from build123d import *

# Parameters (mm, degrees)
F0_R     = 6.5
F0_R_2   = 2.15
F1_DEPTH = 1
F2_R     = 0.49999


# Not quite as in the source:
# - a fillet or chamfer is up to 0.001 mm smaller than in the source, because OpenCascade refuses the exact size


with BuildPart() as f1:
    # F0 (on Top) → F1 (new body)
    with BuildSketch(Plane.XY):
        Circle(F0_R)
        Circle(F0_R_2, mode=Mode.SUBTRACT)
    extrude(amount=F1_DEPTH)

    # F2 (radius 0.5 in the source; OpenCascade refuses exactly that, so slightly less here)
    f2_edges = [f1.edges().sort_by_distance(p)[0] for p in [
        (-6.5, 0, 1),
        (-2.15, 0, 1),
        (6.5, 0, 0.5),
        (-6.5, 0, 0),
        (-2.15, 0, 0),
        (2.15, 0, 0.5),
    ]]
    fillet(f2_edges, radius=F2_R)


solid = f1.part
Can you work these out from the model? Positions are in its coordinate system, mm. Round coordinates to 2 decimals unless told otherwise and drop trailing zeros. Loops run counter-clockwise (first coordinate to the right, second up) from the corner with the lowest first, then second, coordinate; pieces in that order, holes last. Notation, with made-up numbers: (-20, 37) - (-8, 37) arc R21 cw to (-8, 61) - close; hole circle Ø10 at (-28, 54.5). An arc over 180 degrees is marked (long way). Use CSV: the item, a comma, the result in double quotes. Start each with the question number.
1) If we section it at C-C on z = 0.65: Write out the boundary of the cut face in (x, y).
2) Please list where these lines run through material, in increasing order: probe 1 along Y at (x, z) = (0, 0.55); probe 2 along Y at (x, z) = (-1, 0.3); probe 3 along X at (y, z) = (5.25, 0.65). Write a range as [from, to].
3) For pin 1 Ø2 at (x, y) = (2.5, 4.5) entering from -Z, with a flat end and sliding along its axis, tell me the tip position at first contact or that it passes through.
Geometry results:
1,outline,"circle Ø12.95 at (0, 0); hole circle Ø4.35 at (0, 0)"
2,probe 1,"y = [-6.5, -2.15], [2.15, 6.5]"
2,probe 2,"y = [-6.38, -1.95], [1.95, 6.38]"
2,probe 3,"x = [-3.79, 3.79]"
3,pin 1,"stops at z = 0"
